Design review of the part built by this model. Coordinates are the model's own, in mm. A direction names the side the tool comes from. Coordinates: 2 decimals unless noted, no trailing zeros. Write each loop counter-clockwise with the first axis right and the second up, starting at its lowest first coordinate (ties: lowest second). Pieces come first, ordered by that corner, then holes. Notation, with made-up numbers: (-11.75, 30) - (-4.75, 30) arc R18 ccw to (-4.75, 45) - close; hole circle Ø6 at (15, -7). An arc over 180 degrees is marked (long way). Answer as CSV lines item,"result". Start each with the question number.
Q1. For line 1 along Y through (x, z) = (-27, 3.1); line 2 along Y through (x, z) = (-25, 2.7); line 3 along X through (y, z) = (7, 3.2), list the stretches that pass through material, from the lowest coordinate up. Write a range as [from, to].
Q2. We need section D-D (x = 0). Write out the cut boundary in (y, z) (3 decimals), plus the area to 3 significant figures.
Q3. Machinability: for faces 1 (the face through (-27, -6, 2)), 2 (the face through (27, 6, 2)), 3 (the face through (27, -6, 2)), which of the approach directions +Z, -Z, +X, -X, +Y, -Y give a long, thin tool a straight path to every point of the face, cutting with its end or side? Answer none if there is none.
Q4. We need section A-A (z = 1.9). Write out the cut boundary in (x, y) (3 decimals).
Q5. Clearance check with flat-ended pins moving along their axes: pin 1 (1.5 mm diameter, centred on x = 19.5, z = 3, fed in from -Y); pin 2 (0.9 mm diameter, centred on x = -25.5, z = 2.5, fed in from -Y); pin 3 (0.9 mm diameter, centred on x = 27.5, z = 2.5, fed in from +Y); pin 4 (5 mm diameter, centred on x = 27, y = 0, fed in from +Z). State where each tip first meets the part, or that it passes through.
Q6. Mouldability with a two-part tool opening along Y and no side actions: class faces 4 (the face through (-25.5, 0.07, 2.48)), 5 (the face through (-35, 0, 2)), 6 (the face through (28.5, 0.07, 2.48)), 7 (the face through (-27, 6, 2)) as pulls with the +Y half, pulls with the -Y half, needs draft (parallel to the pull), parting line crosses it, or undercut.
Q7. We need section C-C (y = 0). Write out the cut boundary in (x, z) (3 decimals), plus the area to 3 significant figures.
Q8. We need section B-B (x = 27). Write out the cut boundary in (y, z), plus the area to 3 significant figures.
from build123d import *

# Parameters (mm, degrees)
SKETCH2_R           = 20.592109163
SKETCH2_R_2         = 4.125
BOSS_EXTRUDE1_DEPTH = 3
SKETCH3_W           = 70
SKETCH3_H           = 12
SKETCH3_R           = 1.5
SKETCH3_R_2         = 4.125
BOSS_EXTRUDE2_DEPTH = 3


# Read off the part's stored shape, not the designer's step: Gear 60pitch part02.STEP
with BuildPart() as part:
    # Sketch2 → Boss-Extrude1 (new body)
    with BuildSketch(Plane.XY.offset(1)):
        Circle(SKETCH2_R)
        Circle(SKETCH2_R_2, mode=Mode.SUBTRACT)
    extrude(amount=BOSS_EXTRUDE1_DEPTH)

    # Sketch3 → Boss-Extrude2 (add)
    with BuildSketch(Plane(origin=(0, 0, 1), x_dir=(-1, 0, 0), z_dir=(0, 0, -1))):
        Rectangle(SKETCH3_W, SKETCH3_H)
        with Locations((-27, 0)):
            Circle(SKETCH3_R, mode=Mode.SUBTRACT)
        with Locations((27, 0)):
            Circle(SKETCH3_R, mode=Mode.SUBTRACT)
        with Locations(Location((0, 0, 0), (0, 0, 180))):
            Circle(SKETCH3_R_2, mode=Mode.SUBTRACT)
    extrude(amount=-BOSS_EXTRUDE2_DEPTH)


solid = part.part
Results list:
1,line 1,"y = [-6, -1.5], [1.5, 6]"
1,line 2,"y = [-6, 6]"
1,line 3,"x = [-19.37, 19.37]"
2,outline,"(-20.592, 1) - (-4.125, 1) - (-4.125, 4) - (-20.592, 4) - close; (4.125, 1) - (20.592, 1) - (20.592, 4) - (4.125, 4) - close"
2,area,"98.8 mm2"
3,face 1,"+Z, -Z, -X, -Y"
3,face 2,"+Z, -Z, +X, +Y"
3,face 3,"+Z, -Z, +X, -Y"
4,outline,"(-35, -6) - (-19.699, -6) arc R20.592 ccw to (19.699, -6) - (35, -6) - (35, 6) - (19.699, 6) arc R20.592 ccw to (-19.699, 6) - (-35, 6) - close; hole circle Ø3 at (-27, 0); hole circle Ø8.25 at (0, 0); hole circle Ø3 at (27, 0)"
5,pin 1,"stops at y = -8.51"
5,pin 2,"stops at y = -6"
5,pin 3,"stops at y = 6"
5,pin 4,"stops at z = 4"
6,face 4,"undercut"
6,face 5,"needs draft"
6,face 6,"undercut"
6,face 7,"pulls with the +Y half"
7,outline,"(-35, 1) - (-28.5, 1) - (-28.5, 4) - (-35, 4) - close; (-25.5, 1) - (-4.125, 1) - (-4.125, 4) - (-25.5, 4) - close; (4.125, 1) - (25.5, 1) - (25.5, 4) - (4.125, 4) - close; (28.5, 1) - (35, 1) - (35, 4) - (28.5, 4) - close"
7,area,"167 mm2"
8,outline,"(-6, 1) - (-1.5, 1) - (-1.5, 4) - (-6, 4) - close; (1.5, 1) - (6, 1) - (6, 4) - (1.5, 4) - close"
8,area,"27.0 mm2"
